Part model, mm, in its own coordinate system. A direction names the side the tool comes from. Coordinates: 2 decimals unless noted, no trailing zeros. Write each loop counter-clockwise with the first axis right and the second up, starting at its lowest first coordinate (ties: lowest second). Pieces come first, ordered by that corner, then holes. Notation, with made-up numbers: (17.25, -33) - (39.25, -33) arc R17 cw to (39.25, -24) - close; hole circle Ø6 at (29, 75). An arc over 180 degrees is marked (long way). Use one line per item in the form item = value. Start each with the question number.
from build123d import *

# Parameters (mm, degrees)
F0_W     = 381
F0_H     = 88.9
F1_DEPTH = 5.08
F2_W     = 381
F2_H     = 3.81
F3_DEPTH = 12.7
F4_W     = 381
F4_H     = 3.81
F5_DEPTH = 12.7


with BuildPart() as f1:
    # F0 (on Front) → F1 (new body)
    with BuildSketch(Plane.XZ):
        Rectangle(F0_W, F0_H)
    extrude(amount=F1_DEPTH)

    # F2 (on face) → F3 (join)
    with BuildSketch(Plane.XZ.offset(5.08)):
        with Locations((0, 42.545)):
            Rectangle(F2_W, F2_H)
        with Locations((0, -42.545)):
            Rectangle(F2_W, F2_H)
    extrude(amount=F3_DEPTH)

    # F4 (on face) → F5 (join)
    with BuildSketch(Plane.XZ.offset(5.08)):
        with Locations((0, 28.575)):
            Rectangle(F4_W, F4_H)
    extrude(amount=F5_DEPTH)


solid = f1.part
Q1. Slice it at A-A (y = -8). List the corners of the cut face in (x, z).
Q2. Mould opens along Z. For faces 1 (the flat face through (-3, -5.08, -7)), 2 (the flat face through (-3, -11, 40.64)), 3 (the flat face through (190.5, -4.8, 9.3)), 4 (the flat face through (-3, -9, -44.45)) say: released by +Z, released by -Z, zero draft, split by the parting line, or undercut.
Q3. Slice it at B-B (x = 80). List the corners of the cut face in (y, z), plus the area to 3 significant figures.
Q4. Which spindle directions (+Z, -Z, +X, -X, +Y, -Y) get a long thin tool onto all of the face, cutting with end or side? Do faces 5 (the flat face through (-3, -5.08, 36)), 6 (the flat face through (-3, 0, 1)). Say none if no direction does.
Q5. Pin check, flat tip, straight feed: P1, Ø3, axis at x = -7.5, z = 37, coming from the -Y side. Stop position of the tip, or through.
Q6. Drill centre lines: probe 1 along Z at (x, y) = (-39.5, -16.5); probe 2 along Y at (x, z) = (102, 37). Where is each one in solid material? Low to high.
Q7. Slice it at C-C (z = -26). List the corners of the cut face in (x, y), plus the area to 3 significant figures.
Solution:
q1.outline = (-190.5, -44.45) - (190.5, -44.45) - (190.5, -40.64) - (-190.5, -40.64) - close; (-190.5, 26.67) - (190.5, 26.67) - (190.5, 30.48) - (-190.5, 30.48) - close; (-190.5, 40.64) - (190.5, 40.64) - (190.5, 44.45) - (-190.5, 44.45) - close
q2.face_1 = undercut
q2.face_2 = undercut
q2.face_3 = zero draft
q2.face_4 = released by -Z
q3.outline = (-17.78, -44.45) - (0, -44.45) - (0, 44.45) - (-17.78, 44.45) - (-17.78, 40.64) - (-5.08, 40.64) - (-5.08, 30.48) - (-17.78, 30.48) - (-17.78, 26.67) - (-5.08, 26.67) - (-5.08, -40.64) - (-17.78, -40.64) - close
q3.area = 597 mm2
q4.face_5 = +X, -X, -Y
q4.face_6 = +Z, -Z, +X, -X, +Y
q5.P1 = -5.08
q6.probe_1 = -44.45 to -40.64, 26.67 to 30.48, 40.64 to 44.45
q6.probe_2 = -5.08 to 0
q7.outline = (-190.5, -5.08) - (190.5, -5.08) - (190.5, 0) - (-190.5, 0) - close
q7.area = 1,940 mm2
